from build123d import *

# Parameters (mm, degrees)
F1_DEPTH = 1.1
F3_DEPTH = 0.3
F4_DEPTH = 0.3


with BuildPart() as f1:
    # F0 (on Front) → F1 (new body)
    with BuildSketch(Plane.XZ):
        with BuildLine():
            ThreePointArc((1.4361406616, -1), (0.8100925873, -1.5512092057), (0, -1.75))
            Line((0, -1.75), (25, -1.75))
            Line((25, -1.75), (25, -1))
            Line((25, -1), (1.4361406616, -1))
        make_face()
        with BuildLine():
            Line((25, -1), (25, -1.75))
            Line((25, -1.75), (50, -1.75))
            ThreePointArc((50, -1.75), (49.1899074127, -1.5512092057), (48.5638593384, -1))
            Line((48.5638593384, -1), (25, -1))
        make_face()
        with BuildLine():
            Line((48.5638593384, 1), (25, 1))
            Line((25, 1), (25, -1))
            Line((25, -1), (48.5638593384, -1))
            ThreePointArc((48.5638593384, -1), (48.25, 0), (48.5638593384, 1))
        make_face()
        with BuildLine():
            Line((50, 1.75), (25, 1.75))
            Line((25, 1.75), (25, 1))
            Line((25, 1), (48.5638593384, 1))
            ThreePointArc((48.5638593384, 1), (49.1899074127, 1.5512092057), (50, 1.75))
        make_face()
        with BuildLine():
            Line((50, 1), (48.5638593384, 1))
            ThreePointArc((48.5638593384, 1), (48.25, 0), (48.5638593384, -1))
            Line((48.5638593384, -1), (50, -1))
            ThreePointArc((50, -1), (49, 0), (50, 1))
        make_face()
        with BuildLine():
            ThreePointArc((51.75, 0), (51.2374368671, 1.2374368671), (50, 1.75))
            Line((50, 1.75), (50, 1))
            ThreePointArc((50, 1), (50.7071067812, 0.7071067812), (51, 0))
            ThreePointArc((51, 0), (50.7071067812, -0.7071067812), (50, -1))
            Line((50, -1), (50, -1.75))
            ThreePointArc((50, -1.75), (51.2374368671, -1.2374368671), (51.75, 0))
        make_face()
        with BuildLine():
            ThreePointArc((0, -1), (-1, 0), (0, 1))
            Line((0, 1), (0, 1.75))
            ThreePointArc((0, 1.75), (-1.75, 0), (0, -1.75))
            Line((0, -1.75), (0, -1))
        make_face()
        with BuildLine():
            ThreePointArc((0, 1), (0.7071067812, 0.7071067812), (1, 0))
            ThreePointArc((1, 0), (0.7071067812, -0.7071067812), (0, -1))
            Line((0, -1), (1.4361406616, -1))
            ThreePointArc((1.4361406616, -1), (1.6696925103, -0.5240485866), (1.75, 0))
            ThreePointArc((1.75, 0), (1.6696925103, 0.5240485866), (1.4361406616, 1))
            Line((1.4361406616, 1), (0, 1))
        make_face()
        with BuildLine():
            ThreePointArc((48.5638593384, -1), (49.1899074127, -1.5512092057), (50, -1.75))
            Line((50, -1.75), (50, -1))
            Line((50, -1), (48.5638593384, -1))
        make_face()
        with BuildLine():
            Line((50, 1), (50, 1.75))
            ThreePointArc((50, 1.75), (49.1899074127, 1.5512092057), (48.5638593384, 1))
            Line((48.5638593384, 1), (50, 1))
        make_face()
        with BuildLine():
            Line((25, 1), (1.4361406616, 1))
            ThreePointArc((1.4361406616, 1), (1.6696925103, 0.5240485866), (1.75, 0))
            ThreePointArc((1.75, 0), (1.6696925103, -0.5240485866), (1.4361406616, -1))
            Line((1.4361406616, -1), (25, -1))
            Line((25, -1), (25, 1))
        make_face()
        with BuildLine():
            Line((25, 1.75), (0, 1.75))
            ThreePointArc((0, 1.75), (0.8100925873, 1.5512092057), (1.4361406616, 1))
            Line((1.4361406616, 1), (25, 1))
            Line((25, 1), (25, 1.75))
        make_face()
        with BuildLine():
            Line((1.4361406616, -1), (0, -1))
            Line((0, -1), (0, -1.75))
            ThreePointArc((0, -1.75), (0.8100925873, -1.5512092057), (1.4361406616, -1))
        make_face()
        with BuildLine():
            Line((0, 1.75), (0, 1))
            Line((0, 1), (1.4361406616, 1))
            ThreePointArc((1.4361406616, 1), (0.8100925873, 1.5512092057), (0, 1.75))
        make_face()
    extrude(amount=F1_DEPTH)

    # F2 (on face) → F3 (cut)
    with BuildSketch(Plane.XZ.offset(1.1)):
        with BuildLine():
            ThreePointArc((48.5638593384, -1), (48.25, 0), (48.5638593384, 1))
            Line((48.5638593384, 1), (1.4361406616, 1))
            ThreePointArc((1.4361406616, 1), (1.6696925103, 0.5240485866), (1.75, 0))
            ThreePointArc((1.75, 0), (1.6696925103, -0.5240485866), (1.4361406616, -1))
            Line((1.4361406616, -1), (48.5638593384, -1))
        make_face()
    extrude(amount=-F3_DEPTH, mode=Mode.SUBTRACT)

    # F0 (on Front) → F4 (cut)
    with BuildSketch(Plane.XZ):
        with BuildLine():
            Line((48.5638593384, 1), (25, 1))
            Line((25, 1), (25, -1))
            Line((25, -1), (48.5638593384, -1))
            ThreePointArc((48.5638593384, -1), (48.25, 0), (48.5638593384, 1))
        make_face()
        with BuildLine():
            Line((25, 1), (1.4361406616, 1))
            ThreePointArc((1.4361406616, 1), (1.6696925103, 0.5240485866), (1.75, 0))
            ThreePointArc((1.75, 0), (1.6696925103, -0.5240485866), (1.4361406616, -1))
            Line((1.4361406616, -1), (25, -1))
            Line((25, -1), (25, 1))
        make_face()
    extrude(amount=F4_DEPTH, mode=Mode.SUBTRACT)


solid = f1.part
Can you work these out from the model? Positions are in its coordinate system, mm. A direction names the side the tool comes from. Give positions to 0.01 mm unless a question says otherwise; leave off trailing zeros. Loops run counter-clockwise (first coordinate to the right, second up) from the corner with the lowest first, then second, coordinate; pieces in that order, holes last. Notation, with made-up numbers: (-16, 37.25) -> (40, 37.25) arc R22 cw to (40, 49.25) -> close; hole circle Ø6 at (-8, -11). An arc over 180 degrees is marked (long way). Write item = value, one per line.
1) Thinking about a two-plate mould opening in Z: for faces 3 (the flat face through (24.6, -1.1, 1.2)), 4 (the flat face through (24.7, -0.5, -1.75)), 5 (the flat face through (25, -0.8, 0)), 6 (the cylindrical face through (-1.75, -0.54, 0.04)), which applies, released by +Z, released by -Z, zero draft, split by the parting line, or undercut?
Check result:
face_3 = zero draft
face_4 = released by -Z
face_5 = undercut
face_6 = split by the parting line
2) I need wall thicknesses on L1, parallel to X at y = -0.4, z = -0.15; L2, parallel to Z at x = 37.5, y = -0.1; L3, parallel to X at y = -0.9, z = 0.25. Which ranges of each line are inside material? Lowest first, please. Write a range as from..to.
Check result:
L1 = -1.74..-0.99, 0.99..49.01, 50.99..51.74
L2 = -1.75..-1, 1..1.75
L3 = -1.73..-0.97, 0.97..1.73, 48.27..49.03, 50.97..51.73
3) Will this pin go through, and if not, where does the flat tip stop? pin 1 (1 mm diameter, centred on x = 24.5, z = 0, fed in from +Y).
Check result:
pin_1 = -0.3
4) For faces 1 (the flat face through (25, -0.3, 0)), 2 (the flat face through (25.3, -0.5, 1.75)), which set-ups out of +Z, -Z, +X, -X, +Y, -Y let a thin tool reach every point of the face, with its end or its side?
Check result:
face_1 = +Y
face_2 = +Z, +X, -X, +Y, -Y
5) Suppose I cut it at A-A on x = 43. Write out the boundary of the cut face in (y, z), then the cut area to 3 significant figures.
Check result:
outline = (-1.1, -1.75) -> (0, -1.75) -> (0, -1) -> (-0.3, -1) -> (-0.3, 1) -> (0, 1) -> (0, 1.75) -> (-1.1, 1.75) -> (-1.1, 1) -> (-0.8, 1) -> (-0.8, -1) -> (-1.1, -1) -> close
area = 2.65 mm2
